Source: CAD feature listing. Evaluate the final solid. Frame: model axes, mm. A direction names the side the tool comes from. Give positions to 0.01 mm unless a question says otherwise; leave off trailing zeros. Write item = value, one per line.
from build123d import *

# Parameters (mm, degrees)
BOSS_EXTRUDE1_DEPTH = 110
BOSS_EXTRUDE3_DEPTH = 3
LPATTERN1_COUNT     = 15
LPATTERN1_PITCH     = 7


with BuildPart() as part:
    # Sketch2 → Boss-Extrude1 (new body)
    with BuildSketch(Plane(origin=(0, 0, 0), x_dir=(1, 0, 0), z_dir=(0, 1, 0))):
        with BuildLine():
            Line((0, 0), (13, 0))
            ThreePointArc((13, 0), (38, 25), (63, 0))
            Line((63, 0), (78, 0))
            ThreePointArc((78, 0), (103, 25), (128, 0))
            Line((128, 0), (163, 0))
            ThreePointArc((163, 0), (188, 25), (213, 0))
            Line((213, 0), (228, 0))
            ThreePointArc((228, 0), (253, 25), (278, 0))
            Line((278, 0), (291, 0))
            Line((291, 0), (291, 65))
            ThreePointArc((291, 65), (288.071067812, 72.071067812), (281, 75))
            Line((281, 75), (10, 75))
            ThreePointArc((10, 75), (2.928932188, 72.071067812), (0, 65))
            Line((0, 65), (0, 0))
        make_face()
    extrude(amount=BOSS_EXTRUDE1_DEPTH)

    # Sketch4 → Boss-Extrude3 (add)
    with BuildSketch(Plane(origin=(0, 0, 0), x_dir=(1, 0, 0), z_dir=(0, 1, 0))):
        with BuildLine():
            ThreePointArc((10, 75), (2.928932188, 72.071067812), (0, 65))
            Line((0, 65), (0, 0))
            Line((0, 0), (-4, 0))
            Line((-4, 0), (-4, 65))
            ThreePointArc((-4, 65), (0.100505063, 74.899494937), (10, 79))
            Line((10, 79), (281, 79))
            ThreePointArc((281, 79), (290.899494937, 74.899494937), (295, 65))
            Line((295, 65), (295, 0))
            Line((295, 0), (291, 0))
            Line((291, 0), (291, 65))
            ThreePointArc((291, 65), (288.071067812, 72.071067812), (281, 75))
            Line((281, 75), (10, 75))
        make_face()
    boss_extrude3 = extrude(amount=BOSS_EXTRUDE3_DEPTH)

    # LPattern1: Boss-Extrude3 ×15
    with Locations(*[(0, i * LPATTERN1_PITCH, 0) for i in range(1, LPATTERN1_COUNT)]):
        add(boss_extrude3)


solid = part.part
1. Reachability of faces 1 (the cylindrical face through (288.15, 11.97, -71.99)), 2 (the cylindrical face through (3.01, 18.97, -72.15)), 3 (the cylindrical face through (0, 29.5, -74.8)) from +Z, -Z, +X, -X, +Y, -Y: full face, straight path, thin tool, end or side. Return the list, or none.
Derived:
face_1 = -Z, +X
face_2 = -Z, -X
face_3 = -Z, -X, +Y, -Y
2. Material intervals for probe 1 along X at (y, z) = (79.5, -11); probe 2 along X at (y, z) = (45.5, -4); probe 3 along Z at (x, y) = (159, 12.5), sorted ascending. Write a range as from..to.
Derived:
probe_1 = -4..15.55, 60.45..80.55, 125.45..165.55, 210.45..230.55, 275.45..295
probe_2 = 0..13.32, 62.68..78.32, 127.68..163.32, 212.68..228.32, 277.68..291
probe_3 = -75..0
3. First-contact query: pin 1 Ø8 at (x, y) = (116.5, 42.5) entering from +Z; pin 2 Ø2 at (x, y) = (138.5, 81.5) entering from -Z; pin 3 Ø2 at (y, z) = (77.5, -69.5) entering from -X. Flat tips, straight axial feed; report the tip coordinate or a pass-through.
Derived:
pin_1 = -17.85
pin_2 = -75
pin_3 = -3.56
